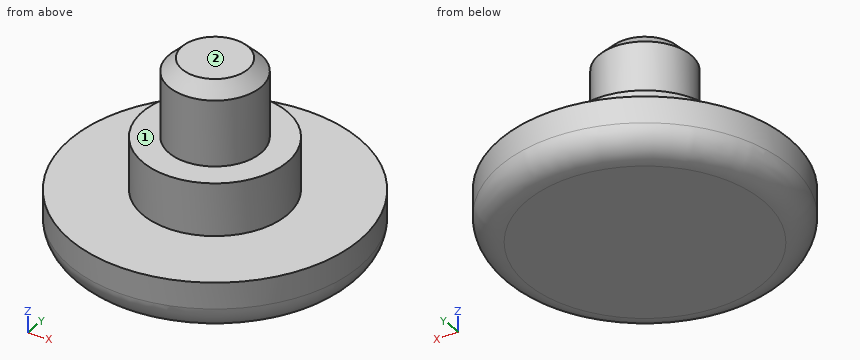
```python
from build123d import *

# Parameters (mm, degrees)
F0_R     = 5.5
F1_DEPTH = 2
F2_R     = 2.75
F3_DEPTH = 2
F4_R     = 1.75
F5_DEPTH = 3
F6_R     = 1
F7_SIZE  = 0.5


with BuildPart() as f1:
    # F0 (on Top) → F1 (new body)
    with BuildSketch(Plane.XY):
        Circle(F0_R)
    extrude(amount=F1_DEPTH)

    # F2 (on face) → F3 (join)
    with BuildSketch(Plane.XY.offset(2)):
        Circle(F2_R)
    extrude(amount=F3_DEPTH)

    # F4 (on face) → F5 (join)
    with BuildSketch(Plane.XY.offset(4)):
        Circle(F4_R)
    extrude(amount=F5_DEPTH)

    # F6
    f6_edges = [f1.edges().sort_by_distance(p)[0] for p in [
        (-5.5, 0, 0),
    ]]
    fillet(f6_edges, radius=F6_R)

    # F7
    f7_edges = [f1.edges().sort_by_distance(p)[0] for p in [
        (-1.75, 0, 7),
    ]]
    chamfer(f7_edges, length=F7_SIZE)


solid = f1.part
```
Verification items for the finished model (mm, model axes). Face numbers are marked on the shaded views. A direction names the side the tool comes from. Coordinates: 2 decimals unless noted, no trailing zeros. Order: outer loops, then holes, each group sorted by start corner. A loop starts at its lowest first (then second) coordinate and runs counter-clockwise, first axis right, second up. Notation, with made-up numbers: (-9.75, -5.75) -> (13.25, -5.75) arc R33 ccw to (13.25, 22.25) -> close; hole circle Ø9 at (-28, 41.5). An arc over 180 degrees is marked (long way). Put each result on its own line as item: value. Start each with the question number.
1) Go/stop test with flat-tipped pins: pin 1 (4 mm diameter, centred on y = 2.5, z = 3.5, fed in from +X); pin 2 (1 mm diameter, centred on x = 2.5, z = 2, fed in from -Y); pin 3 (3 mm diameter, centred on x = -1, y = 1, fed in from +Z); pin 4 (2 mm diameter, centred on x = -1.5, z = 3.5, fed in from -Y). Record where each tip stops, or that it passes through.
2) Material ranges on L1, parallel to Z at x = -2.5, y = -1.25; L2, parallel to X at y = -2.25, z = 1.5; L3, parallel to Y at x = -2, z = 0.75, recorded low to high.
3) Tool access check on the marked faces 1 and 2. Record the directions out of +Z, -Z, +X, -X, +Y, -Y that give a thin tool (end or side, any length) a straight path to the whole face; none if there is none.
4) Cross-section at C-C (z = 4.25). Enter the section's corners in (x, y).
5) Cross-section at A-A (y = 0). Enter the section's corners in (x, z), plus the area to 3 significant figures.
Geometry check:
1. pin 1: stops at x = 5.37
1. pin 2: stops at y = -5.12
1. pin 3: stops at z = 7
1. pin 4: stops at y = -2.7
2. L1: z = 0 to 2
2. L2: x = -5.02 to 5.02
2. L3: y = -5.09 to 5.09
3. face 1: +Z
3. face 2: +Z, +X, -X, +Y, -Y
4. outline: circle Ø3.5 at (0, 0)
5. outline: (-5.5, 1) arc R1 ccw to (-4.5, 0) -> (4.5, 0) arc R1 ccw to (5.5, 1) -> (5.5, 2) -> (2.75, 2) -> (2.75, 4) -> (1.75, 4) -> (1.75, 6.5) -> (1.25, 7) -> (-1.25, 7) -> (-1.75, 6.5) -> (-1.75, 4) -> (-2.75, 4) -> (-2.75, 2) -> (-5.5, 2) -> close
5. area: 42.8 mm^2
